Model file for the job. Use its own axes, mm. Face numbers are marked on the shaded views. A direction names the side the tool comes from. Coordinates: 2 decimals unless noted, no trailing zeros. Order: outer loops, then holes, each group sorted by start corner. A loop starts at its lowest first (then second) coordinate and runs counter-clockwise, first axis right, second up.
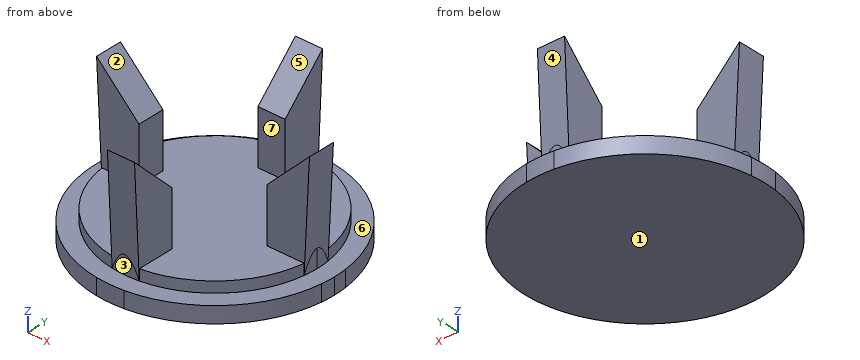
from build123d import *

# Parameters (mm, degrees)
F1_DEPTH     = 1.5
F2_DEPTH     = 10
F4_DEPTH     = 2.5
F6_DEPTH     = 2.5
F8_DEPTH     = 2.5
F10_DEPTH    = 2.5
F11_DEPTH    = 1
F12_T1_DEPTH = 23.0734639037
F12_T3_DEPTH = 23.0734639037


# Not quite as in the source:
# - a fillet or chamfer that OpenCascade refuses, or shapes differently, is made with other operations: its cross-section is extruded or revolved along the edge and cut away or added


with BuildPart() as f1:
    # F0 (on Top) → F1 (new body)
    with BuildSketch(Plane.XY):
        with BuildLine():
            Line((-1.25, 9.3165175897), (-1.25, 10.9287464972))
            ThreePointArc((-1.25, 10.9287464972), (-7.7781745931, 7.7781745931), (-10.9287464972, 1.25))
            Line((-10.9287464972, 1.25), (-9.3165175897, 1.25))
            ThreePointArc((-9.3165175897, 1.25), (-6.6468037432, 6.6468037432), (-1.25, 9.3165175897))
        make_face()
        with BuildLine():
            ThreePointArc((-10.9287464972, -1.25), (-7.7781745931, -7.7781745931), (-1.25, -10.9287464972))
            Line((-1.25, -10.9287464972), (-1.25, -9.3165175897))
            ThreePointArc((-1.25, -9.3165175897), (-6.6468037432, -6.6468037432), (-9.3165175897, -1.25))
            Line((-9.3165175897, -1.25), (-10.9287464972, -1.25))
        make_face()
        with BuildLine():
            Line((-9.3165175897, 1.25), (-10.9287464972, 1.25))
            ThreePointArc((-10.9287464972, 1.25), (-11, 0), (-10.9287464972, -1.25))
            Line((-10.9287464972, -1.25), (-9.3165175897, -1.25))
            ThreePointArc((-9.3165175897, -1.25), (-9.4, 0), (-9.3165175897, 1.25))
        make_face()
        with BuildLine():
            ThreePointArc((1.25, -10.9287464972), (7.7781745931, -7.7781745931), (10.9287464972, -1.25))
            Line((10.9287464972, -1.25), (9.3165175897, -1.25))
            ThreePointArc((9.3165175897, -1.25), (6.6468037432, -6.6468037432), (1.25, -9.3165175897))
            Line((1.25, -9.3165175897), (1.25, -10.9287464972))
        make_face()
        with BuildLine():
            ThreePointArc((-1.25, -10.9287464972), (0, -11), (1.25, -10.9287464972))
            Line((1.25, -10.9287464972), (1.25, -9.3165175897))
            ThreePointArc((1.25, -9.3165175897), (0, -9.4), (-1.25, -9.3165175897))
            Line((-1.25, -9.3165175897), (-1.25, -10.9287464972))
        make_face()
        with BuildLine():
            Line((9.3165175897, 1.25), (10.9287464972, 1.25))
            ThreePointArc((10.9287464972, 1.25), (7.7781745931, 7.7781745931), (1.25, 10.9287464972))
            Line((1.25, 10.9287464972), (1.25, 9.3165175897))
            ThreePointArc((1.25, 9.3165175897), (6.6468037432, 6.6468037432), (9.3165175897, 1.25))
        make_face()
        with BuildLine():
            ThreePointArc((10.9287464972, -1.25), (10.9821721774, -0.6260145888), (11, 0))
            ThreePointArc((11, 0), (10.9821721774, 0.6260145888), (10.9287464972, 1.25))
            Line((10.9287464972, 1.25), (9.3165175897, 1.25))
            ThreePointArc((9.3165175897, 1.25), (9.3791061766, 0.6263923117), (9.4, 0))
            ThreePointArc((9.4, 0), (9.3791061766, -0.6263923117), (9.3165175897, -1.25))
            Line((9.3165175897, -1.25), (10.9287464972, -1.25))
        make_face()
        with BuildLine():
            Line((1.25, 9.3165175897), (1.25, 10.9287464972))
            ThreePointArc((1.25, 10.9287464972), (0, 11), (-1.25, 10.9287464972))
            Line((-1.25, 10.9287464972), (-1.25, 9.3165175897))
            ThreePointArc((-1.25, 9.3165175897), (0, 9.4), (1.25, 9.3165175897))
        make_face()
        with BuildLine():
            Line((5.9, 1.25), (9.3165175897, 1.25))
            ThreePointArc((9.3165175897, 1.25), (6.6468037432, 6.6468037432), (1.25, 9.3165175897))
            Line((1.25, 9.3165175897), (1.25, 5.9))
            Line((1.25, 5.9), (-1.25, 5.9))
            Line((-1.25, 5.9), (-1.25, 9.3165175897))
            ThreePointArc((-1.25, 9.3165175897), (-6.6468037432, 6.6468037432), (-9.3165175897, 1.25))
            Line((-9.3165175897, 1.25), (-5.9, 1.25))
            Line((-5.9, 1.25), (-5.9, -1.25))
            Line((-5.9, -1.25), (-9.3165175897, -1.25))
            ThreePointArc((-9.3165175897, -1.25), (-6.6468037432, -6.6468037432), (-1.25, -9.3165175897))
            Line((-1.25, -9.3165175897), (-1.25, -5.9))
            Line((-1.25, -5.9), (1.25, -5.9))
            Line((1.25, -5.9), (1.25, -9.3165175897))
            ThreePointArc((1.25, -9.3165175897), (6.6468037432, -6.6468037432), (9.3165175897, -1.25))
            Line((9.3165175897, -1.25), (5.9, -1.25))
            Line((5.9, -1.25), (5.9, 1.25))
        make_face()
        with BuildLine():
            Line((1.25, 5.9), (1.25, 9.3165175897))
            ThreePointArc((1.25, 9.3165175897), (0, 9.4), (-1.25, 9.3165175897))
            Line((-1.25, 9.3165175897), (-1.25, 5.9))
            Line((-1.25, 5.9), (1.25, 5.9))
        make_face()
        with BuildLine():
            ThreePointArc((9.4, 0), (9.3791061766, 0.6263923117), (9.3165175897, 1.25))
            Line((9.3165175897, 1.25), (5.9, 1.25))
            Line((5.9, 1.25), (5.9, -1.25))
            Line((5.9, -1.25), (9.3165175897, -1.25))
            ThreePointArc((9.3165175897, -1.25), (9.3791061766, -0.6263923117), (9.4, 0))
        make_face()
        with BuildLine():
            Line((-5.9, 1.25), (-9.3165175897, 1.25))
            ThreePointArc((-9.3165175897, 1.25), (-9.4, 0), (-9.3165175897, -1.25))
            Line((-9.3165175897, -1.25), (-5.9, -1.25))
            Line((-5.9, -1.25), (-5.9, 1.25))
        make_face()
        with BuildLine():
            ThreePointArc((-1.25, -9.3165175897), (0, -9.4), (1.25, -9.3165175897))
            Line((1.25, -9.3165175897), (1.25, -5.9))
            Line((1.25, -5.9), (-1.25, -5.9))
            Line((-1.25, -5.9), (-1.25, -9.3165175897))
        make_face()
    extrude(amount=-F1_DEPTH)

    # F0 (on Top) → F2 (join)
    with BuildSketch(Plane.XY):
        with BuildLine():
            Line((1.25, 5.9), (1.25, 9.3165175897))
            ThreePointArc((1.25, 9.3165175897), (0, 9.4), (-1.25, 9.3165175897))
            Line((-1.25, 9.3165175897), (-1.25, 5.9))
            Line((-1.25, 5.9), (1.25, 5.9))
        make_face()
        with BuildLine():
            ThreePointArc((9.4, 0), (9.3791061766, 0.6263923117), (9.3165175897, 1.25))
            Line((9.3165175897, 1.25), (5.9, 1.25))
            Line((5.9, 1.25), (5.9, -1.25))
            Line((5.9, -1.25), (9.3165175897, -1.25))
            ThreePointArc((9.3165175897, -1.25), (9.3791061766, -0.6263923117), (9.4, 0))
        make_face()
        with BuildLine():
            Line((-5.9, 1.25), (-9.3165175897, 1.25))
            ThreePointArc((-9.3165175897, 1.25), (-9.4, 0), (-9.3165175897, -1.25))
            Line((-9.3165175897, -1.25), (-5.9, -1.25))
            Line((-5.9, -1.25), (-5.9, 1.25))
        make_face()
        with BuildLine():
            ThreePointArc((-1.25, -9.3165175897), (0, -9.4), (1.25, -9.3165175897))
            Line((1.25, -9.3165175897), (1.25, -5.9))
            Line((1.25, -5.9), (-1.25, -5.9))
            Line((-1.25, -5.9), (-1.25, -9.3165175897))
        make_face()
    extrude(amount=F2_DEPTH)

    # F3 (on face) → F4 (join)
    with BuildSketch(Plane(origin=(-1.25, 0, 0), x_dir=(0, -1, 0), z_dir=(-1, 0, 0))):
        Polygon((-9.3165175897, 0), (-9.3165175897, 10), (-9.8165175897, 10), align=None)
    extrude(amount=-F4_DEPTH)

    # F5 (on face) → F6 (join)
    with BuildSketch(Plane(origin=(-1.25, 0, 0), x_dir=(0, -1, 0), z_dir=(-1, 0, 0))):
        Polygon((9.8165175897, 10), (9.3165175897, 10), (9.3165175897, 0), align=None)
    extrude(amount=-F6_DEPTH)

    # F7 (on face) → F8 (join)
    with BuildSketch(Plane.XZ.offset(1.25)):
        Polygon((-9.3165175897, 0), (-9.3165175897, 10), (-9.8165175897, 10), align=None)
    extrude(amount=-F8_DEPTH)

    # F9 (on face) → F10 (join)
    with BuildSketch(Plane.XZ.offset(1.25)):
        Polygon((9.8165175897, 10), (9.3165175897, 10), (9.3165175897, 0), align=None)
    extrude(amount=-F10_DEPTH)

    # F0 (on Top) → F11 (join)
    with BuildSketch(Plane.XY):
        with BuildLine():
            Line((5.9, 1.25), (9.3165175897, 1.25))
            ThreePointArc((9.3165175897, 1.25), (6.6468037432, 6.6468037432), (1.25, 9.3165175897))
            Line((1.25, 9.3165175897), (1.25, 5.9))
            Line((1.25, 5.9), (-1.25, 5.9))
            Line((-1.25, 5.9), (-1.25, 9.3165175897))
            ThreePointArc((-1.25, 9.3165175897), (-6.6468037432, 6.6468037432), (-9.3165175897, 1.25))
            Line((-9.3165175897, 1.25), (-5.9, 1.25))
            Line((-5.9, 1.25), (-5.9, -1.25))
            Line((-5.9, -1.25), (-9.3165175897, -1.25))
            ThreePointArc((-9.3165175897, -1.25), (-6.6468037432, -6.6468037432), (-1.25, -9.3165175897))
            Line((-1.25, -9.3165175897), (-1.25, -5.9))
            Line((-1.25, -5.9), (1.25, -5.9))
            Line((1.25, -5.9), (1.25, -9.3165175897))
            ThreePointArc((1.25, -9.3165175897), (6.6468037432, -6.6468037432), (9.3165175897, -1.25))
            Line((9.3165175897, -1.25), (5.9, -1.25))
            Line((5.9, -1.25), (5.9, 1.25))
        make_face()
    extrude(amount=F11_DEPTH)

    # F12: chamfer of 4 on 4 edges, made by hand

    # F12_s2 → F12_t1 (cut)
    with BuildSketch(Plane.YZ.offset(-11.5367319519)):
        Polygon((5.9, 6), (9.9, 10), (5.9, 10), align=None)
        Polygon((-9.9, 10), (-5.9, 6), (-5.9, 10), align=None)
    extrude(amount=F12_T1_DEPTH, mode=Mode.SUBTRACT)

    # F12_s4 → F12_t3 (cut)
    with BuildSketch(Plane.XZ.offset(-11.5367319519)):
        Polygon((9.9, 10), (5.9, 6), (5.9, 10), align=None)
        Polygon((-5.9, 6), (-9.9, 10), (-5.9, 10), align=None)
    extrude(amount=F12_T3_DEPTH, mode=Mode.SUBTRACT)


solid = f1.part
Q1. Cut at C-C, the plane x = -4.5. List the corners of the cut face in (y, z).
Established:
outline: (-10.04, -1.5) - (10.04, -1.5) - (10.04, 0) - (8.25, 0) - (8.25, 1) - (-8.25, 1) - (-8.25, 0) - (-10.04, 0) - close
Q2. Cut at A-A, the plane z = 8.5. List the corners of the cut face in (x, y).
Established:
outline: (-9.74, -1.25) - (-8.4, -1.25) - (-8.4, 1.25) - (-9.74, 1.25) - close; (-1.25, -9.74) - (1.25, -9.74) - (1.25, -8.4) - (-1.25, -8.4) - close; (-1.25, 8.4) - (1.25, 8.4) - (1.25, 9.74) - (-1.25, 9.74) - close; (8.4, -1.25) - (9.74, -1.25) - (9.74, 1.25) - (8.4, 1.25) - close
Q3. Mould opens along Y. For the marked faces 4, 5, 6 and 7 say: pulls with the +Y half, pulls with the -Y half, needs draft (parallel to the pull), parting line crosses it, or undercut.
Established:
face 4: pulls with the +Y half
face 5: undercut
face 6: needs draft
face 7: undercut
Q4. Which spindle directions (+Z, -Z, +X, -X, +Y, -Y) get a long thin tool onto all of the face, cutting with end or side? Do the marked faces 1, 2 and 3. Say none if no direction does.
Established:
face 1: -Z, +X, -X, +Y, -Y
face 2: +Z, +Y, -Y
face 3: -Y
Q5. Probe line 1 (Z direction, x = 1.5, y = 7.75); line 2 (X direction, y = 8, z = 5.5); line 3 (X direction, y = 0, z = 2.25). List the from-to ranges inside material, lowest first.
Established:
line 1: z = -1.5 to 1
line 2: x = -1.25 to 1.25
line 3: x = -9.43 to -5.9, 5.9 to 9.43
Q6. Drop flat-ended pins along their axis: P1, Ø1.2, axis at y = -8.5, z = 7, coming from the +X side; P2, Ø5, axis at x = 7, z = 8, coming from the -Y side; P3, Ø4, axis at y = -6.5, z = 8.5, coming from the -X side. Give the stop position or say it passes through.
Established:
P1: stops at x = 1.25
P2: stops at y = -1.25
P3: stops at x = -1.25
Q7. Cut at B-B, the plane y = -5.5. List the corners of the cut face in (x, z).
Established:
outline: (-9.53, -1.5) - (9.53, -1.5) - (9.53, 0) - (7.62, 0) - (7.62, 1) - (-7.62, 1) - (-7.62, 0) - (-9.53, 0) - close
Q8. Cut at D-D, the plane z = 3.75. List the corners of the cut face in (x, y), plus the area to 3 significant figures.
Established:
outline: (-9.5, -1.25) - (-5.9, -1.25) - (-5.9, 1.25) - (-9.5, 1.25) - close; (-1.25, -9.5) - (1.25, -9.5) - (1.25, -5.9) - (-1.25, -5.9) - close; (-1.25, 5.9) - (1.25, 5.9) - (1.25, 9.5) - (-1.25, 9.5) - close; (5.9, -1.25) - (9.5, -1.25) - (9.5, 1.25) - (5.9, 1.25) - close
area: 36.0 mm2
